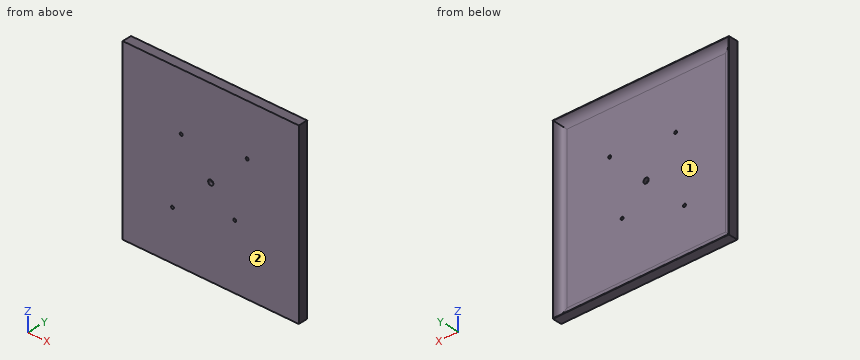
```python
from build123d import *

# Parameters (mm, degrees)
SKETCH_1_W      = 200
SKETCH_1_H      = 200
SKETCH_1_R      = 3
SKETCH_1_R_2    = 1.65
EXTRUDE_1_DEPTH = 4
EXTRUDE_3_DEPTH = 100
EXTRUDE_4_DEPTH = 100


with BuildPart() as part:
    # 草图1 → 凸台-拉伸1 (new body)
    with BuildSketch(Plane(origin=(0, 0, 0), x_dir=(1, 0, 0), z_dir=(0, 1, 0))):
        Rectangle(SKETCH_1_W, SKETCH_1_H)
        with Locations(Location((0, 0, 0), (0, 0, 270))):
            Circle(SKETCH_1_R, mode=Mode.SUBTRACT)
        with Locations(Location((27.223611076, 26.516504294, 0), (0, 0, 270))):
            Circle(SKETCH_1_R_2, mode=Mode.SUBTRACT)
        with Locations(Location((-43.487067043, 43.487067043, 0), (0, 0, 270))):
            Circle(SKETCH_1_R_2, mode=Mode.SUBTRACT)
        with Locations(Location((-33.587572106, -34.294678888, 0), (0, 0, 270))):
            Circle(SKETCH_1_R_2, mode=Mode.SUBTRACT)
        with Locations(Location((41.365746699, -41.365746699, 0), (0, 0, 270))):
            Circle(SKETCH_1_R_2, mode=Mode.SUBTRACT)
    extrude(amount=EXTRUDE_1_DEPTH)

    # 草图3 → 凸台-拉伸3 (add, symmetric)
    with BuildSketch(Plane(origin=(0, 0, 0), x_dir=(0, 0, -1), z_dir=(1, 0, 0))):
        with BuildLine():
            Line((-100, 4), (-90, 4))
            ThreePointArc((-90, 4), (-95.760553163, 5.825892877), (-99.417475728, 10.636794548))
            ThreePointArc((-99.417475728, 10.636794548), (-99.751199211, 10.831497168), (-100, 10.535898385))
            Line((-100, 10.535898385), (-100, 4))
        make_face()
        with BuildLine():
            Line((100, 4), (100, 10.535898385))
            ThreePointArc((100, 10.535898385), (99.751199211, 10.831497168), (99.417475728, 10.636794548))
            ThreePointArc((99.417475728, 10.636794548), (95.760553163, 5.825892877), (90, 4))
            Line((90, 4), (100, 4))
        make_face()
    extrude(amount=EXTRUDE_3_DEPTH, both=True)

    # 草图5 → 凸台-拉伸4 (add, symmetric)
    with BuildSketch(Plane.XY):
        with BuildLine():
            Line((-100, 4), (-90, 4))
            ThreePointArc((-90, 4), (-95.760553163, 5.825892877), (-99.417475728, 10.636794548))
            ThreePointArc((-99.417475728, 10.636794548), (-99.751199211, 10.831497168), (-100, 10.535898385))
            Line((-100, 10.535898385), (-100, 4))
        make_face()
        with BuildLine():
            Line((100, 4), (100, 10.535898385))
            ThreePointArc((100, 10.535898385), (99.751199211, 10.831497168), (99.417475728, 10.636794548))
            ThreePointArc((99.417475728, 10.636794548), (95.760553163, 5.825892877), (90, 4))
            Line((90, 4), (100, 4))
        make_face()
    extrude(amount=EXTRUDE_4_DEPTH, both=True)


solid = part.part
```
Can you work these out from the model? Positions are in its coordinate system, mm. Face numbers are marked on the shaded views. Give positions to 0.01 mm unless a question says otherwise; leave off trailing zeros. Order: outer loops, then holes, each group sorted by start corner. A loop starts at its lowest first (then second) coordinate and runs counter-clockwise, first axis right, second up. Notation, with made-up numbers: (44, 22) - (98, 22) arc R26 cw to (98, 45) - close; hole circle Ø2 at (11.5, 50.25). An arc over 180 degrees is marked (long way). Use a Markdown table: item, result. Add a question column.
Q1. If we section it at B-B on x = 0: Write out the boundary of the cut face in (y, z).
Q2. If we section it at D-D on x = -25: Write out the boundary of the cut face in (y, z), plus the area to 3 significant figures.
Q3. I'm going to push flat-ended pins straight in: pin 1 (5 mm diameter, centred on x = 53, z = -15, fed in from -Y); pin 2 (8 mm diameter, centred on x = 0, z = 0, fed in from +Y). Where does each tip first touch, or does it pass through?
Q4. If we section it at A-A on z = 0: Write out the boundary of the cut face in (x, y).
Q5. Please list where these lines run through material, in increasing order: line 1 along Z through (x, y) = (84, 6.75); line 2 along Z through (x, y) = (60, 5).
Q6. If we section it at C-C on y = 7.75: Write out the boundary of the cut face in (x, z), plus the area to 3 significant figures.
Q7. If we mould it in two halves opening along Z, with no side actions, what happens to the marked faces 1 and 2? For each: released by +Z, released by -Z, zero draft, split by the parting line, or undercut.
Answers follow:
| question | item | result |
|---|---|---|
| 1 | outline | (0, -100) - (10.54, -100) arc R0.3 ccw to (10.64, -99.42) arc R10 cw to (4, -90) - (4, -3) - (0, -3) - close; (0, 3) - (4, 3) - (4, 90) arc R10 cw to (10.64, 99.42) arc R0.3 ccw to (10.54, 100) - (0, 100) - close |
| 2 | outline | (0, -100) - (10.54, -100) arc R0.3 ccw to (10.64, -99.42) arc R10 cw to (4, -90) - (4, 90) arc R10 cw to (10.64, 99.42) arc R0.3 ccw to (10.54, 100) - (0, 100) - close |
| 2 | area | 842 mm^2 |
| 3 | pin 1 | stops at y = 0 |
| 3 | pin 2 | stops at y = 4 |
| 4 | outline | (-100, 0) - (-3, 0) - (-3, 4) - (-90, 4) arc R10 cw to (-99.42, 10.64) arc R0.3 ccw to (-100, 10.54) - close; (3, 0) - (100, 0) - (100, 10.54) arc R0.3 ccw to (99.42, 10.64) arc R10 cw to (90, 4) - (3, 4) - close |
| 5 | line 1 | z = -100 to -96.89, 96.89 to 100 |
| 5 | line 2 | z = -100 to -94.36, 94.36 to 100 |
| 6 | outline | (-100, -100) - (100, -100) - (100, 100) - (-100, 100) - close; hole (-97.81, -97.81) - (97.81, -97.81) - (97.81, 97.81) - (-97.81, 97.81) - close |
| 6 | area | 1,740 mm^2 |
| 7 | face 1 | undercut |
| 7 | face 2 | zero draft |
